```python
from build123d import *

# Parameters (mm, degrees)
SKETCH1_W           = 25
SKETCH1_H           = 52
BOSS_EXTRUDE1_DEPTH = 7
SKETCH2_R           = 1
CUT_EXTRUDE1_DEPTH  = 30.685855218
LPATTERN1_COUNT     = 6
LPATTERN1_PITCH     = 8
SKETCH9_R           = 1.65
SKETCH9_R_2         = 1.6
CUT_EXTRUDE3_DEPTH  = 4.25
LPATTERN2_COUNT     = 6
LPATTERN2_PITCH     = 8
CHAMFER2_SIZE       = 4
SKETCH10_W          = 14.9
SKETCH10_H          = 52
CUT_EXTRUDE4_DEPTH  = 2
CHAMFER3_SIZE       = 2
BOSS_EXTRUDE2_DEPTH = 3
BOSS_EXTRUDE3_DEPTH = 4
SKETCH13_R          = 1.65
CUT_EXTRUDE5_DEPTH  = 3
CUT_EXTRUDE6_REACH  = 31.686
SKETCH14_R          = 3


# Some blends are built 0.0001 mm under size
with BuildPart() as part:
    # Sketch1 → Boss-Extrude1 (new body)
    with BuildSketch(Plane(origin=(0, 0, 0), x_dir=(1, 0, 0), z_dir=(0, 1, 0))):
        Rectangle(SKETCH1_W, SKETCH1_H)
    extrude(amount=BOSS_EXTRUDE1_DEPTH)

    # Sketch2 → Cut-Extrude1 (cut, through all)
    with BuildSketch(Plane(origin=(0, 7, 0), x_dir=(1, 0, 0), z_dir=(0, 1, 0))):
        with Locations(Location((-10.45, -20, 0), (0, 0, 270))):
            Circle(SKETCH2_R)
        with Locations(Location((10.45, -20, 0), (0, 0, 270))):
            Circle(SKETCH2_R)
    cut_extrude1 = extrude(amount=-CUT_EXTRUDE1_DEPTH, mode=Mode.SUBTRACT)

    # LPattern1: Cut-Extrude1 ×6
    with Locations(*[(0, 0, -i * LPATTERN1_PITCH) for i in range(1, LPATTERN1_COUNT)]):
        add(cut_extrude1, mode=Mode.SUBTRACT)

    # Sketch9 → Cut-Extrude3 (cut)
    with BuildSketch(Plane(origin=(0, 7, 0), x_dir=(1, 0, 0), z_dir=(0, 1, 0))):
        with Locations(Location((-10.45, 20, 0), (0, 0, 270))):
            Circle(SKETCH9_R)
        with Locations(Location((10.45, 20, 0), (0, 0, 270))):
            Circle(SKETCH9_R_2)
    cut_extrude3 = extrude(amount=-CUT_EXTRUDE3_DEPTH, mode=Mode.SUBTRACT)

    # LPattern2: Cut-Extrude3 ×6
    with Locations(*[(0, 0, i * LPATTERN2_PITCH) for i in range(1, LPATTERN2_COUNT)]):
        add(cut_extrude3, mode=Mode.SUBTRACT)

    # Chamfer2
    # the kernel refuses this chamfer: 4 mm, written as the material it takes off along each edge
    with BuildSketch(Plane(origin=(-12.5, 7, -36.286731952), x_dir=(-0.027495876610586487, -0.9996219169112968, 0), z_dir=(0, 0, 1)), Plane(origin=(12.5, 7, 36.286731952), x_dir=(0.027495876610586487, -0.9996219169112968, 0), z_dir=(0, 0, -1))) as chamfer2_piece_1:
        Polygon((CHAMFER2_SIZE * 0.999621916911, CHAMFER2_SIZE * 0.0274958766106), (-CHAMFER2_SIZE * 0.0274958766106, CHAMFER2_SIZE * 0.999621916911), (0, 0), align=None)
    extrude(amount=72.573463904, mode=Mode.SUBTRACT)

    # Sketch10 → Cut-Extrude4 (cut)
    with BuildSketch(Plane.XZ):
        Rectangle(SKETCH10_W, SKETCH10_H)
    extrude(amount=-CUT_EXTRUDE4_DEPTH, mode=Mode.SUBTRACT)

    # Chamfer3
    chamfer3_edges = [part.edges().sort_by_distance(p)[0] for p in [
        (7.45, 2, 0),
        (-7.45, 2, 0),
    ]]
    chamfer(chamfer3_edges, length=CHAMFER3_SIZE - 0.0001)  # a hair under: the kernel refuses the full size

    # Sketch12 → Boss-Extrude2 (add)
    with BuildSketch(Plane(origin=(0, 7, 0), x_dir=(1, 0, 0), z_dir=(0, 1, 0))):
        with BuildLine():
            ThreePointArc((8.5, 5.728219619), (0, 10.25), (-8.5, 5.728219619))
            Line((-8.5, 5.728219619), (-8.5, -5.728219619))
            ThreePointArc((-8.5, -5.728219619), (0, -10.25), (8.5, -5.728219619))
            Line((8.5, -5.728219619), (8.5, 5.728219619))
        make_face()
    extrude(amount=BOSS_EXTRUDE2_DEPTH)

    # Sketch12<3> → Boss-Extrude3 (add)
    with BuildSketch(Plane(origin=(0, 7, 0), x_dir=(1, 0, 0), z_dir=(0, 1, 0))):
        with BuildLine():
            ThreePointArc((8.5, 10.164275675), (0, 13.25), (-8.5, 10.164275675))
            Line((-8.5, 10.164275675), (-8.5, 5.728219619))
            ThreePointArc((-8.5, 5.728219619), (0, 10.25), (8.5, 5.728219619))
            Line((8.5, 5.728219619), (8.5, 10.164275675))
        make_face()
        with BuildLine():
            Line((-8.5, -5.728219619), (-8.5, -10.164275675))
            ThreePointArc((-8.5, -10.164275675), (0, -13.25), (8.5, -10.164275675))
            Line((8.5, -10.164275675), (8.5, -5.728219619))
            ThreePointArc((8.5, -5.728219619), (0, -10.25), (-8.5, -5.728219619))
        make_face()
    extrude(amount=BOSS_EXTRUDE3_DEPTH)

    # Sketch13 → Cut-Extrude5 (cut)
    with BuildSketch(Plane(origin=(0, 10, 0), x_dir=(1, 0, 0), z_dir=(0, 1, 0))):
        with Locations(Location((-4.949747468, 4.949747468, 0), (0, 0, 270))):
            Circle(SKETCH13_R)
        with Locations(Location((4.949747468, 4.949747468, 0), (0, 0, 270))):
            Circle(SKETCH13_R)
        with Locations(Location((4.949747468, -4.949747468, 0), (0, 0, 270))):
            Circle(SKETCH13_R)
        with Locations(Location((-4.949747468, -4.949747468, 0), (0, 0, 270))):
            Circle(SKETCH13_R)
        with Locations(Location((0, 0, 0), (0, 0, 270))):
            Circle(SKETCH13_R)
    extrude(amount=-CUT_EXTRUDE5_DEPTH, mode=Mode.SUBTRACT)

    # Sketch14 → Cut-Extrude6 (cut, up to next)
    with BuildSketch(Plane(origin=(0, 7, 0), x_dir=(1, 0, 0), z_dir=(0, 1, 0)), mode=Mode.PRIVATE) as cut_extrude6_sk1:
        with Locations(Location((-4.949747468, 4.949747468, 0), (0, 0, 270))):
            Circle(SKETCH14_R)
    cut_extrude6_tool1 = extrude(cut_extrude6_sk1.sketch, amount=-CUT_EXTRUDE6_REACH, mode=Mode.PRIVATE) & part.part
    # Sketch14 → Cut-Extrude6 (cut, up to next)
    with BuildSketch(Plane(origin=(0, 7, 0), x_dir=(1, 0, 0), z_dir=(0, 1, 0)), mode=Mode.PRIVATE) as cut_extrude6_sk2:
        with Locations(Location((4.949747468, 4.949747468, 0), (0, 0, 270))):
            Circle(SKETCH14_R)
    cut_extrude6_tool2 = extrude(cut_extrude6_sk2.sketch, amount=-CUT_EXTRUDE6_REACH, mode=Mode.PRIVATE) & part.part
    # Sketch14 → Cut-Extrude6 (cut, up to next)
    with BuildSketch(Plane(origin=(0, 7, 0), x_dir=(1, 0, 0), z_dir=(0, 1, 0)), mode=Mode.PRIVATE) as cut_extrude6_sk3:
        with Locations(Location((4.949747468, -4.949747468, 0), (0, 0, 270))):
            Circle(SKETCH14_R)
    cut_extrude6_tool3 = extrude(cut_extrude6_sk3.sketch, amount=-CUT_EXTRUDE6_REACH, mode=Mode.PRIVATE) & part.part
    # Sketch14 → Cut-Extrude6 (cut, up to next)
    with BuildSketch(Plane(origin=(0, 7, 0), x_dir=(1, 0, 0), z_dir=(0, 1, 0)), mode=Mode.PRIVATE) as cut_extrude6_sk4:
        with Locations(Location((-4.949747468, -4.949747468, 0), (0, 0, 270))):
            Circle(SKETCH14_R)
    cut_extrude6_tool4 = extrude(cut_extrude6_sk4.sketch, amount=-CUT_EXTRUDE6_REACH, mode=Mode.PRIVATE) & part.part
    # Sketch14 → Cut-Extrude6 (cut, up to next)
    with BuildSketch(Plane(origin=(0, 7, 0), x_dir=(1, 0, 0), z_dir=(0, 1, 0)), mode=Mode.PRIVATE) as cut_extrude6_sk5:
        with Locations(Location((0, 0, 0), (0, 0, 270))):
            Circle(SKETCH14_R)
    cut_extrude6_tool5 = extrude(cut_extrude6_sk5.sketch, amount=-CUT_EXTRUDE6_REACH, mode=Mode.PRIVATE) & part.part
    add(cut_extrude6_tool1.solids().sort_by_distance((-4.949747, 7, -4.949747))[0], mode=Mode.SUBTRACT)
    add(cut_extrude6_tool2.solids().sort_by_distance((4.949747, 7, -4.949747))[0], mode=Mode.SUBTRACT)
    add(cut_extrude6_tool3.solids().sort_by_distance((4.949747, 7, 4.949747))[0], mode=Mode.SUBTRACT)
    add(cut_extrude6_tool4.solids().sort_by_distance((-4.949747, 7, 4.949747))[0], mode=Mode.SUBTRACT)
    add(cut_extrude6_tool5.solids().sort_by_distance((0, 7, 0))[0], mode=Mode.SUBTRACT)


solid = part.part
```
Source: CAD feature listing. Evaluate the final solid. Frame: model axes, mm. A direction names the side the tool comes from. Give positions to 0.01 mm unless a question says otherwise; leave off trailing zeros.
1. Section query A-A (y = 1.25). Count the separate pieces of the cut face and the enclosed holes in it, then the cut area to 3 significant figures.
2. Pull-direction query (Z, two-part tool) for faces 4 (the face through (-11.06, 1.39, -20.79)), 5 (the face through (10.5, 5, 0.4)); classes: +Z half, -Z half, draft (parallel to the pull), parting line (faces both ways), or undercut.
3. First-contact query: pin 1 (3.5 mm diameter, centred on x = 0, z = 0, fed in from -Y); pin 2 (5.5 mm diameter, centred on x = 4.95, z = -4.95, fed in from +Y); pin 3 (1.6 mm diameter, centred on x = -10.5, z = -21, fed in from +Y); pin 4 (1.9 mm diameter, centred on x = 10.45, z = 20, fed in from +Y). Flat tips, straight axial feed; report the tip coordinate or a pass-through.
4. Access query for faces 1 (the face through (7.924, 4.327, 4.559)), 2 (the face through (-8.814, 4.314, -4.215)), 3 (the face through (6.46, 0.99, 16.17)). Directions: +Z, -Z, +X, -X, +Y, -Y. A direction counts if a zero-diameter tool reaches every point of the face in a straight line with its end or side. Return the directions, or none.
5. Material intervals for line 1 along X through (y, z) = (1.8, 12); line 2 along X through (y, z) = (7.8, 0); line 3 along Y through (x, z) = (1.5, -18.5), sorted ascending.
Output values:
1. separate pieces: 2
1. enclosed holes: 12
1. area: 590 mm2
2. face 4: undercut
2. face 5: draft
3. pin 1: stops at y = 7
3. pin 2: stops at y = 10
3. pin 3: stops at y = 5.56
3. pin 4: passes through
4. face 1: -Y
4. face 2: +Y
4. face 3: +Z, -Z, -Y
5. line 1: x = -12.5 to -11.45, -9.45 to -5.65, 5.65 to 9.45, 11.45 to 12.5
5. line 2: x = -8.5 to -1.65, 1.65 to 8.5
5. line 3: y = 2 to 7
